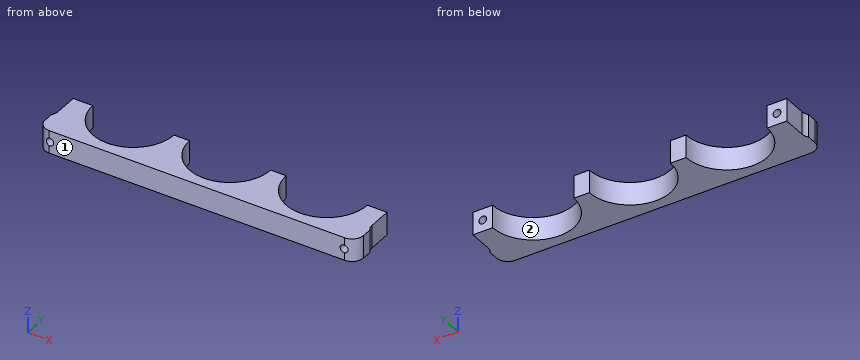
Autodesk Inventor part; units mm, degrees
ref_plane "YZ Plane" through (0, 0, 0) normal (1, 0, 0) x (0, 1, 0)
ref_plane "XZ Plane" through (0, 0, 0) normal (0, 1, 0) x (-1, 0, 0)
ref_plane "XY Plane" through (0, 0, 0) normal (0, 0, 1) x (1, 0, 0)
sketch "Sketch1" plane through (0, 0, 0) normal (0, 0, 1) x (1, 0, 0)
  line L0 (-44.323, 14.2875) -> (44.323, 14.2875)
  line L1 (44.323, 14.2875) -> (44.323, -14.2875)
  line L2 (44.323, -14.2875) -> (-44.323, -14.2875)
  line L3 (-44.323, -14.2875) -> (-44.323, 14.2875)
  point P0 (0, 0)
  dimension "d0" = 88.646
  dimension "d1" = 44.323
  dimension "d2" = 14.2875
  dimension "d3" = 28.575
extrude "Extrusion1" add sketch "Sketch1" along normal mid plane 6.35
sketch "Sketch2" plane through (0, 0, 3.175) normal (0, 0, 1) x (1, 0, 0)
  circle A0 centre (-26.924, 0) radius 11.303
  circle A1 centre (0, 0) radius 11.303
  line L0 (44.323, -14.2875) -> (44.323, 14.2875)
  circle A2 centre (26.924, 0) radius 11.303
  line L1 (-44.323, 14.2875) -> (-44.323, -14.2875)
  line L2 (-44.323, 0) -> (44.323, 0) construction
  line L3 (44.323, 14.2875) -> (-44.323, 14.2875)
  point P0 (0, 0)
  dimension "d6" = 22.606
  dimension "d9" = 22.606
  dimension "d11" = 22.606
  dimension "d14" = 26.924
  dimension "d21" = 88.646
  dimension "d22" = 26.924
  dimension "d50" = 0
sketch "Sketch4" plane through (-44.323, -14.2875, -3.175) normal (-1, 0, 0) x (0, 0, 1)
  line L0 (0, 0) -> (0, 28.575)
  line L1 (6.35, 28.575) -> (6.35, 0)
  line L2 (0, 22.6695) -> (6.35, 22.6695)
  line L3 (6.35, 22.6695) -> (6.35, 5.9055)
  line L4 (6.35, 5.9055) -> (0, 5.9055)
  line L5 (0, 5.9055) -> (0, 22.6695)
  point P0 (3.175, 14.2875)
  dimension "d30" = 8.382
  dimension "d31" = 16.764
extrude "Extrusion3" cut sketch "Sketch4" against normal blind 0.635
mirror "Mirror1" about plane through (0, 0, 0) normal (1, 0, 0) of "Extrusion3"
sketch "Sketch7" plane through (-44.323, -14.2875, 3.175) normal (0, -1, 0) x (1, 0, 0)
  line L0 (30.353, -14.605) -> (58.293, -14.605)
  line L1 (58.293, -14.605) -> (58.293, 8.255)
  line L2 (58.293, 8.255) -> (30.353, 8.255)
  line L3 (30.353, 8.255) -> (30.353, -14.605)
  point P0 (44.323, -3.175)
  dimension "d39" = 27.94
  dimension "d40" = 22.86
  dimension "d41" = 11.43
  dimension "d42" = 13.97
extrude "Extrusion5" [suppressed]
sketch "Sketch8" plane through (0, 0, -3.175) normal (0, 0, -1) x (-1, 0, 0)
  line L0 (-44.323, 14.2875) -> (44.323, 14.2875)
  line L1 (15.6718, 14.2875) -> (-15.6718, 14.2875)
  line L2 (-15.6718, 14.2875) -> (-15.6718, 52.3875)
  line L3 (-15.6718, 52.3875) -> (15.6718, 52.3875)
  line L4 (15.6718, 52.3875) -> (15.6718, 14.2875)
  point P0 (0, 0)
  dimension "d45" = 31.3436
  dimension "d46" = 38.1
  dimension "d47" = 15.6718
extrude "Extrusion6" add sketch "Sketch8" against normal up to surface (6.35 mm away)
extrude "Extrusion7" cut sketch "Sketch2" against normal blind 25.4
sketch "Sketch9" plane through (-15.6718, 52.3875, -3.175) normal (0, 1, 0) x (1, 0, 0)
  line L0 (-28.6512, -6.35) -> (59.9948, -6.35)
  line L1 (3.1718, -6.35) -> (28.1718, -6.35)
  line L2 (28.1718, -6.35) -> (28.1718, -3.175)
  line L3 (28.1718, -3.175) -> (3.1718, -3.175)
  line L4 (3.1718, -3.175) -> (3.1718, -6.35)
  point P0 (15.6718, -3.175)
  dimension "d64" = 3.175
  dimension "d65" = 25
  dimension "d66" = 12.5
extrude "Extrusion8" cut sketch "Sketch9" against normal blind 0.9
sketch "Sketch13" plane through (0, 0, 3.175) normal (0, 0, 1) x (1, 0, 0)
  line L0 (-15.6718, 52.3875) -> (-12.5, 52.3875)
  line L1 (-12.5, 52.3875) -> (12.5, 52.3875)
  line L2 (12.5, 52.3875) -> (15.6718, 52.3875)
  line L3 (15.6718, 52.3875) -> (15.6718, 14.2875)
  line L4 (-15.6718, 14.2875) -> (-15.6718, 52.3875)
  line L5 (-15.6718, 14.2875) -> (-44.323, 14.2875)
  line L6 (44.323, 14.2875) -> (15.6718, 14.2875)
  line L7 (44.323, 8.382) -> (44.323, 14.2875)
  line L8 (-44.323, 14.2875) -> (-44.323, 8.382)
  line L9 (-44.323, 8.382) -> (-43.688, 8.382)
  line L10 (43.688, 8.382) -> (44.323, 8.382)
  line L11 (-43.688, 8.382) -> (-43.688, 0)
  line L12 (-43.688, 8.382) -> (-43.688, -8.382)
  line L13 (-43.688, 0) -> (43.688, 0)
  line L14 (43.688, 8.382) -> (43.688, -8.382)
  line L15 (43.688, 0) -> (43.688, 8.382)
  point P0 (0, 0)
extrude "Extrusion11" cut sketch "Sketch13" against normal through all
fillet "Fillet3" radius 3.175 2 edges at (-43.688, -8.382, 0) (43.688, -8.382, 0)
fillet "Fillet1" radius 3.175 2 edges at (44.323, -14.2875, 0) (-44.323, -14.2875, 0)
sketch "Sketch14" plane through (-43.688, 0, 3.175) normal (0, 1, 0) x (1, 0, 0)
  line L0 (5.461, 6.35) -> (5.461, 0)
  line L1 (0, 6.35) -> (5.461, 6.35)
  line L2 (0, 0) -> (0, 6.35)
  line L3 (5.461, 0) -> (0, 0)
  circle A0 centre (2.7305, 3.175) radius 1.5494
  point P0 (43.688, 3.175)
  dimension "d84" = 3.0988
  dimension "d85" = 5.461
  dimension "d87" = 3.175
  dimension "d88" = 2.7305
  dimension "d98" = 6.35
hole "Hole1" at (-40.9575, 0, 0) direction (0, -1, 0) diameter 2.159 end through all
mirror "Mirror4" about plane through (0, 0, 0) normal (1, 0, 0) of "Hole1"
equation "\"d9\" = d7"
equation "\"d11\" = d9"
equation "\"d22\" = d14"
equation "\"d87\" = 0.5 * d98"
equation "\"d88\" = 0.5 * d85"
equation "\"d7\" = d6"
properties part number "Tube Holder Halve 3" material "Aluminum 6061-AHC"
Part model, mm, in its own coordinate system. Face numbers are marked on the shaded views. Coordinates: 2 decimals unless noted, no trailing zeros. Write each loop counter-clockwise with the first axis right and the second up, starting at its lowest first coordinate (ties: lowest second). Pieces come first, ordered by that corner, then holes. Notation, with made-up numbers: M 61,-32.75 L 116,-32.75 A20 cw 116,-27.75 Z; hole C 85.5,17.25 d3. An arc over 180 degrees is marked long. Return JSON: item names as keys, results as strings.
1. Pull direction X, two halves, no side cores. Call the marked faces 1 and 2: pulls with the +X half, pulls with the -X half, needs draft (parallel to the pull), parting line crosses it, or undercut.
Determined:
{"face 1": "needs draft", "face 2": "undercut"}
2. Saw through at C-C, the plane x = 0. Write the cut outline in (y, z) (1 decimal), then the cut area to 3 significant figures.
Determined:
{"outline": "M -14.3,-3.2 L -11.3,-3.2 L -11.3,3.2 L -14.3,3.2 Z", "area": "19.0 mm²"}
3. Saw through at A-A, the plane y = -4. Write the cut outline in (x, z) (1 decimal), then the cut area to 3 significant figures.
Determined:
{"outline": "M -43.7,-3.2 L -37.5,-3.2 L -37.5,3.2 L -43.7,3.2 Z; M -16.4,-3.2 L -10.6,-3.2 L -10.6,3.2 L -16.4,3.2 Z; M 10.6,-3.2 L 16.4,-3.2 L 16.4,3.2 L 10.6,3.2 Z; M 37.5,-3.2 L 43.7,-3.2 L 43.7,3.2 L 37.5,3.2 Z; hole C -41,0 d2.2; hole C 41,0 d2.2", "area": "145 mm²"}
4. Saw through at B-B, the plane z = 0. Count the separate pieces of the cut face and the enclosed holes in it, then the cut area to 3 significant figures.
Determined:
{"separate pieces": "3", "enclosed holes": "0", "area": "589 mm²"}
5. Saw through at D-D, the plane x = -34. Write the cut outline in (y, z) (1 decimal), then the cut area to 3 significant figures.
Determined:
{"outline": "M -14.3,-3.2 L -8.8,-3.2 L -8.8,3.2 L -14.3,3.2 Z", "area": "34.8 mm²"}
6. Flat gauge pins, fed straight in: pin 1 Ø2 at (y, z) = (-6.5, 0) entering from +X; pin 2 Ø4 at (x, y) = (21, -7) entering from +Z. Where does each tip first touch, or does it go through?
Determined:
{"pin 1": "x = 43.86", "pin 2": "through"}
7. Probe L1, parallel to X at y = -6.75, z = 0; L2, parallel to X at y = -9.5, z = -0.5; L3, parallel to X at y = -8.25, z = -1.25. List the from-to ranges inside material, lowest first.
Determined:
{"L1": "-43.7 to -42.04, -39.88 to -35.99, -17.86 to -9.07, 9.07 to 17.86, 35.99 to 39.88, 42.04 to 43.7", "L2": "-44.32 to -41.91, -40 to -33.05, -20.8 to -6.12, 6.12 to 20.8, 33.05 to 40, 41.91 to 44.32", "L3": "-44.23 to -34.65, -19.2 to -7.73, 7.73 to 19.2, 34.65 to 44.23"}
